Input: part model. Units: mm. Frame: model coordinates. A direction names the side the tool comes from. Round coordinates to 2 decimals unless told otherwise and drop trailing zeros. Loops run counter-clockwise (first coordinate to the right, second up) from the corner with the lowest first, then second, coordinate; pieces in that order, holes last. Notation, with made-up numbers: M -38,50.5 L -19,50.5 A17 cw -19,76.5 Z; hole C 41,-37 d6. An arc over 180 degrees is marked long. Return JSON: item names as keys, results as strings. Group by question number.
1) Section C-C (z = 9.25). Output: boundary loops of the cut face in (x, y), plus the area to 3 significant figures.
2) Section D-D (x = -8). Output: boundary loops of the cut face in (y, z).
3) Section B-B (z = 25). Output: boundary loops of the cut face in (x, y), plus the area to 3 significant figures.
4) Material intervals for line 1 (X direction, y = 12, z = 26.75); line 2 (Y direction, x = 9, z = 20.5); line 3 (Y direction, x = 18.5, z = 4), sorted ascending. Write a range as from..to.
5) Contact query for flat-ended pins moving along their axis: P1, Ø10, axis at x = 22, y = -20, coming from the +Z side; P2, Ø1.5, axis at y = -14.5, z = 4, coming from the +X side; P3, Ø0.6, axis at y = -27, z = 5, coming from the +X side. Output: stop coordinate, or through.
6) Section A-A (y = -25.5). Output: boundary loops of the cut face in (x, z).
7) Access query for faces 5 (the face through (-1, -30.5, 15)), 6 (the face through (47.5, 0, 18)), 7 (the face through (24, -18, 2)). Directions: +Z, -Z, +X, -X, +Y, -Y. A direction counts if a zero-diameter tool reaches every point of the face in a straight line with its end or side. Return the directions, or none.
8) Mould query, pull axis X, two halves, no side actions, for faces 1 (the face through (-1, 30.5, 15)), 2 (the face through (-1, 28, 18)), 3 (the face through (50, 0, 15)), 4 (the face through (-50, 0, 15)). Classes: +X half, -X half, draft (parallel to the pull), parting line (faces both ways), or undercut.
from build123d import *

# Parameters (mm, degrees)
SKETCH022_W     = 100
SKETCH022_H     = 61
PAD013_DEPTH    = 30
SKETCH023_W     = 95
SKETCH023_H     = 56
POCKET004_DEPTH = 25
SKETCH024_W     = 20
SKETCH024_H     = 9.5
POCKET005_DEPTH = 2.5
SKETCH025_W     = 20
SKETCH025_H     = 2.5
POCKET006_DEPTH = 50
SKETCH026_W     = 17
SKETCH026_H     = 0.5
POCKET007_DEPTH = 50


with BuildPart() as part:
    # Sketch022 → Pad013 (new body)
    with BuildSketch(Plane.XY):
        Rectangle(SKETCH022_W, SKETCH022_H)
    extrude(amount=PAD013_DEPTH)

    # Sketch023 (on Face6 of Pad013) → Pocket004 (cut)
    with BuildSketch(Plane.XY.offset(30)):
        Rectangle(SKETCH023_W, SKETCH023_H)
    extrude(amount=-POCKET004_DEPTH, mode=Mode.SUBTRACT)

    # Sketch024 (on Face3 of Pocket004) → Pocket005 (cut)
    with BuildSketch(Plane.YZ.offset(50)):
        with Locations((-18, 6.75)):
            Rectangle(SKETCH024_W, SKETCH024_H)
    extrude(amount=-POCKET005_DEPTH, mode=Mode.SUBTRACT)

    # Sketch025 (on Face13 of Pocket005) → Pocket006 (cut)
    with BuildSketch(Plane.YZ.offset(47.5)):
        with Locations((-18, 3.25)):
            Rectangle(SKETCH025_W, SKETCH025_H)
    extrude(amount=-POCKET006_DEPTH, mode=Mode.SUBTRACT)

    # Sketch026 (on Face1 of Pocket006) → Pocket007 (cut)
    with BuildSketch(Plane.YZ.offset(47.5)):
        with Locations((-18, 4.75)):
            Rectangle(SKETCH026_W, SKETCH026_H)
    extrude(amount=-POCKET007_DEPTH, mode=Mode.SUBTRACT)


solid = part.part
Returned:
{
 "1": {"outline": "M -50,-30.5 L 50,-30.5 L 50,-28 L -47.5,-28 L -47.5,28 L 47.5,28 L 47.5,-8 L 50,-8 L 50,30.5 L -50,30.5 Z", "area": "730 mm^2"},
 "2": {"outline": "M -30.5,0 L 30.5,0 L 30.5,30 L 28,30 L 28,5 L -28,5 L -28,30 L -30.5,30 Z"},
 "3": {"outline": "M -50,-30.5 L 50,-30.5 L 50,30.5 L -50,30.5 Z; hole M -47.5,-28 L 47.5,-28 L 47.5,28 L -47.5,28 Z", "area": "780 mm^2"},
 "4": {"line 1": "x = -50..-47.5, 47.5..50", "line 2": "y = -30.5..-28, 28..30.5", "line 3": "y = -30.5..-28, -8..30.5"},
 "5": {"P1": "stops at z = 2", "P2": "stops at x = -2.5", "P3": "stops at x = 47.5"},
 "6": {"outline": "M -50,0 L 50,0 L 50,2 L -2.5,2 L -2.5,5 L -47.5,5 L -47.5,30 L -50,30 Z; M 47.5,11.5 L 50,11.5 L 50,30 L 47.5,30 Z"},
 "7": {"face 5": "+Z, -Z, +X, -X, -Y", "face 6": "+Z", "face 7": "+X"},
 "8": {"face 1": "draft", "face 2": "undercut", "face 3": "+X half", "face 4": "-X half"}
}
